Geometry check sheet. Reference: drawing and pictorial views, mm from the part's lowest x, y, z. A direction names the side the tool comes from. Round coordinates to 2 decimals unless told otherwise and drop trailing zeros. Loops run counter-clockwise (first coordinate to the right, second up) from the corner with the lowest first, then second, coordinate; pieces in that order, holes last. Notation, with made-up numbers: (87.25, -26.75) -> (143.25, -26.75) arc R18 ccw to (143.25, 8.25) -> close; hole circle Ø5 at (-21.5, -13.75). An arc over 180 degrees is marked (long way). Use one line per item in the form item = value. Start each with the question number.
(1) Draft check along X on the marked faces 1, 2 and 3. Enter one of: released by +X, released by -X, zero draft, split by the parting line, or undercut.
(2) Sectioned sample at B-B (y = 8.25). Record the cut outline in (x, z).
(3) Set-up check for the marked faces 4, 5 and 6: record each of +Z, -Z, +X, -X, +Y, -Y from which the full face is reachable in a straight line by a thin tool's end or side.
(4) Sectioned sample at D-D (x = 20). Record the cut outline in (y, z), and give its area (4 significant figures).
(5) Material ranges on probe 1 along Z at (x, y) = (10.5, 2.25); probe 2 along Y at (x, z) = (17.25, 0.9) (3 decimals); probe 3 along Y at (x, z) = (5.25, 1.45) (3 decimals), recorded low to high. Write a range as [from, to].
(6) Sectioned sample at A-A (x = 17.25). Record the cut outline in (y, z) (3 decimals), and give its area (4 significant figures).
(7) Sectioned sample at C-C (z = 4.75). Record the cut outline in (x, y).
(8) Go/stop test with flat-tipped pins: pin 1 (1.3 mm diameter, centred on y = 4.5, z = 14.5, fed in from +X); pin 2 (12 mm diameter, centred on x = 13.5, z = 5, fed in from +Y); pin 3 (1.3 mm diameter, centred on y = 5, z = 11.5, fed in from -X); pin 4 (2 mm diameter, centred on x = 7.5, y = 3, fed in from +Z). Record where each tip stops, or that it passes through.
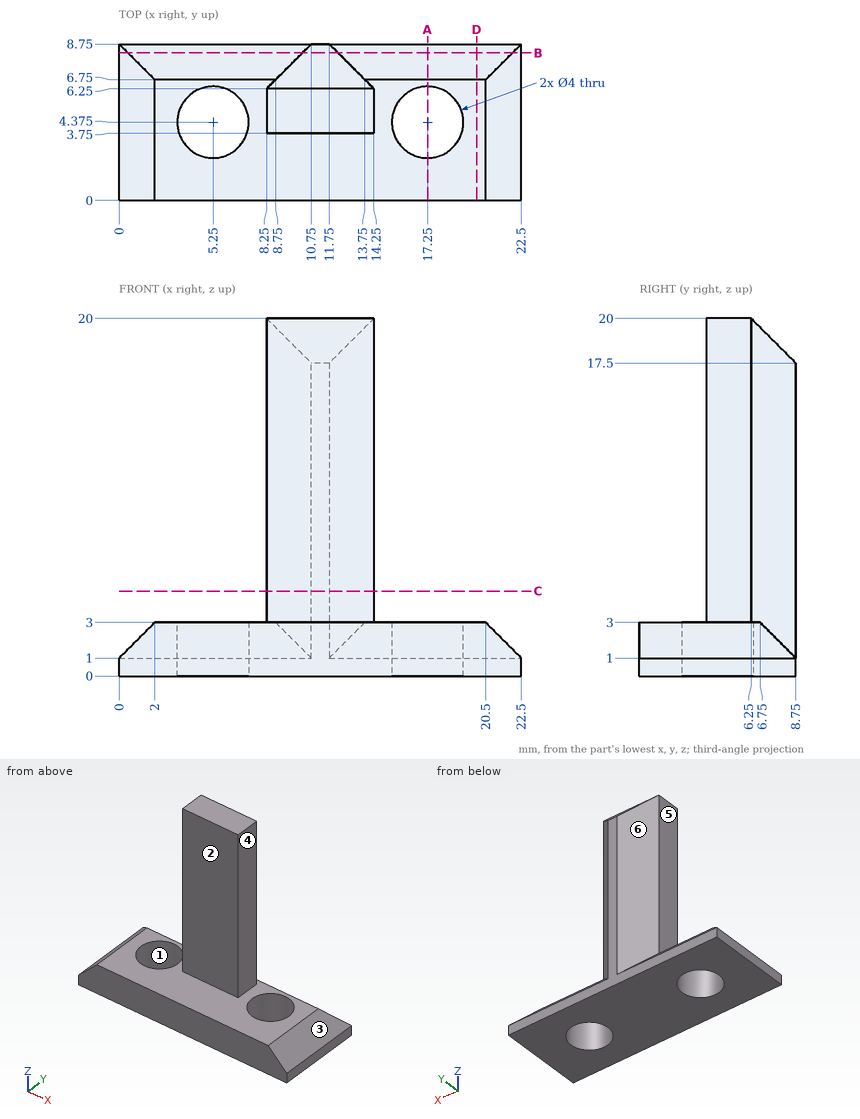
Checks:
q1.face_1 = undercut
q1.face_2 = zero draft
q1.face_3 = released by +X
q2.outline = (0, 0) -> (22.5, 0) -> (22.5, 1) -> (22, 1.5) -> (12.25, 1.5) -> (12.25, 18) -> (10.25, 18) -> (10.25, 1.5) -> (0.5, 1.5) -> (0, 1) -> close
q3.face_4 = +Z, +X, +Y, -Y
q3.face_5 = +Z, -X, +Y, -Y
q3.face_6 = +Z, -X, +Y
q4.outline = (0, 0) -> (8.75, 0) -> (8.75, 1) -> (6.75, 3) -> (0, 3) -> close
q4.area = 24.25 mm2
q5.probe_1 = [0, 3]
q5.probe_2 = [0, 2.375], [6.375, 8.75]
q5.probe_3 = [0, 2.375], [6.375, 8.3]
q6.outline = (0, 0) -> (2.375, 0) -> (2.375, 3) -> (0, 3) -> close; (6.375, 0) -> (8.75, 0) -> (8.75, 1) -> (6.75, 3) -> (6.375, 3) -> close
q6.area = 12.25 mm2
q7.outline = (8.25, 3.75) -> (14.25, 3.75) -> (14.25, 6.25) -> (11.75, 8.75) -> (10.75, 8.75) -> (8.25, 6.25) -> close
q8.pin_1 = 14.25
q8.pin_2 = 8.75
q8.pin_3 = 8.25
q8.pin_4 = 3
